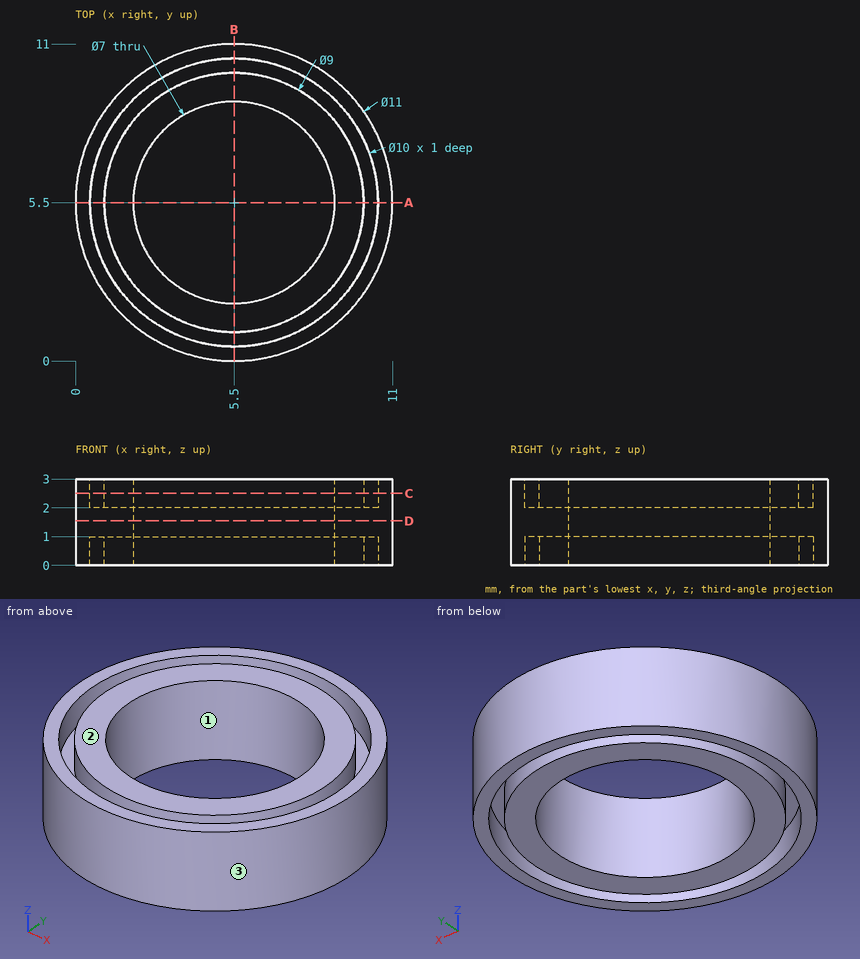
Could you check a few things on this drawing? It's one solid part, dimensions in mm from its lowest x, y, z. Coordinates: 2 decimals unless noted, no trailing zeros. Order: outer loops, then holes, each group sorted by start corner. A loop starts at its lowest first (then second) coordinate and runs counter-clockwise, first axis right, second up. Notation, with made-up numbers: M -10,77.25 L 42,77.25 A13 ccw 42,96.25 Z; hole C 20.5,30 d3. An arc over 180 degrees is marked long. Use a Markdown table: item, result. Add a question column.
Q1. We'd pull the mould along Y, two halves only. Please class the marked faces 1, 2 and 3: pulls with the +Y half, pulls with the -Y half, needs draft (parallel to the pull), parting line crosses it, or undercut.
Q2. If I drill on L1, parallel to Y at x = 5.5, z = 2.3; L2, parallel to X at y = 9.5, z = 0.2; L3, parallel to X at y = 4.25, z = 0.9, over which ranges is the centre line in solid material (lowest first)?
Q3. I want a section at D-D on z = 1.55. List the corners of the cut face in (x, y) for me, then the cut area to 3 significant figures.
Q4. I want a section at A-A on y = 5.5. List the corners of the cut face in (x, z) for me, then the cut area to 3 significant figures.
Q5. I want a section at C-C on z = 2.5. List the corners of the cut face in (x, y) for me.
Q6. I'm going to push flat-ended pins straight in: pin 1 (6 mm diameter, centred on x = 6.5, y = 5.5, fed in from +Z); pin 2 (1.5 mm diameter, centred on y = 3.5, z = 2.5, fed in from -X). Where does each tip first touch, or does it pass through?
Checked values:
| question | item | result |
|---|---|---|
| 1 | face 1 | undercut |
| 1 | face 2 | needs draft |
| 1 | face 3 | parting line crosses it |
| 2 | L1 | 0 to 0.5, 1 to 2, 9 to 10, 10.5 to 11 |
| 2 | L2 | 1.73 to 2.5, 3.44 to 7.56, 8.5 to 9.27 |
| 2 | L3 | 0.14 to 0.66, 1.18 to 2.23, 8.77 to 9.82, 10.34 to 10.86 |
| 3 | outline | C 5.5,5.5 d11; hole C 5.5,5.5 d7 |
| 3 | area | 56.5 mm² |
| 4 | outline | M 0,0 L 0.5,0 L 0.5,1 L 1,1 L 1,0 L 2,0 L 2,3 L 1,3 L 1,2 L 0.5,2 L 0.5,3 L 0,3 Z; M 9,0 L 10,0 L 10,1 L 10.5,1 L 10.5,0 L 11,0 L 11,3 L 10.5,3 L 10.5,2 L 10,2 L 10,3 L 9,3 Z |
| 4 | area | 10.0 mm² |
| 5 | outline | C 5.5,5.5 d11; C 5.5,5.5 d9; hole C 5.5,5.5 d10; hole C 5.5,5.5 d7 |
| 6 | pin 1 | z = 3 |
| 6 | pin 2 | x = 0.14 |
